Source: CAD feature listing. Evaluate the final solid. Frame: model axes, mm. Face numbers are marked on the shaded views. A direction names the side the tool comes from. Round coordinates to 2 decimals unless told otherwise and drop trailing zeros. Loops run counter-clockwise (first coordinate to the right, second up) from the corner with the lowest first, then second, coordinate; pieces in that order, holes last. Notation, with made-up numbers: (78.5, -1.75) -> (130.5, -1.75) arc R34 cw to (130.5, 28.25) -> close; hole circle Ø5 at (2, -6). An arc over 180 degrees is marked (long way). Write item = value, one per line.
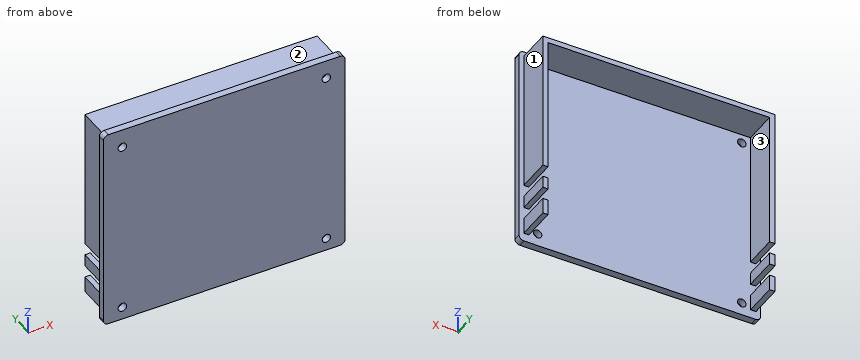
Autodesk Inventor part; units mm, degrees
ref_plane "YZ Plane" through (0, 0, 0) normal (1, 0, 0) x (0, 1, 0)
ref_plane "XZ Plane" through (0, 0, 0) normal (0, 1, 0) x (-1, 0, 0)
ref_plane "XY Plane" through (0, 0, 0) normal (0, 0, 1) x (1, 0, 0)
sketch "Sketch1" plane through (0, 0, 0) normal (0, 1, 0) x (-1, 0, 0)
  line L0 (0, 0) -> (100, 0)
  line L1 (100, 0) -> (100, -85)
  line L2 (100, -85) -> (0, -85)
  line L3 (0, -85) -> (0, 0)
  line L4 (100, -85) -> (100, -81.5)
  line L5 (100, -85) -> (0, -85)
  line L6 (0, 0) -> (100, 0)
  dimension "d0" = 100
  dimension "d1" = 85
extrude "Extrusion1" add sketch "Sketch1" along normal blind 3
sketch "Sketch5" plane through (0, 3, 0) normal (0, 1, 0) x (1, 0, 0)
  line L0 (-100, 85.001914) -> (0, 85.001914)
  line L1 (0, 85.001914) -> (0, 0.001914)
  line L2 (0, 0.001914) -> (-100, 0.001914)
  line L3 (0, 0.001914) -> (0, 3.501877)
  line L4 (0, 0.001914) -> (-100, 0.001914)
  line L5 (-100, 85.001914) -> (0, 85.001914)
  line L6 (-100, 85) -> (-100, 0)
  line L7 (-100, 85) -> (-100, 0)
  line L8 (0, 81.501879) -> (-13.977379, 81.501879)
  line L9 (0, 85) -> (-100, 85)
  line L10 (-13.977379, 81.501879) -> (-13.977379, 85)
  line L11 (0, 0) -> (0, 85)
  line L12 (0, 81.501879) -> (0, 85)
  line L13 (0, 85) -> (-13.977379, 85)
  line L14 (0, 81.501879) -> (-6, 81.501879)
  line L15 (-100, 85) -> (-100, 0)
  line L16 (-100, 0) -> (0, 0)
  line L17 (-100, 81.501917) -> (-84.168275, 81.501917)
  line L18 (-84.168275, 85) -> (-84.168275, 81.501917)
  line L19 (-93.931804, 81.467894) -> (-95.682804, 81.467894)
  line L20 (-98.248671, 81.501917) -> (-100, 81.501917)
  line L21 (-47.950989, 85) -> (-11.964435, 85)
  line L22 (-57.205258, 85) -> (-86.408023, 85)
  circle A0 centre (-7.75, 7.751877) radius 1.75
  circle A1 centre (-92.181804, 7.751877) radius 1.75
  circle A2 centre (-7.724421, 79.777458) radius 1.724421
  circle A3 centre (-92.171647, 79.74176) radius 1.760157
  line L23 (-6, 6.035046) -> (-6, 6.001877)
  line L24 (-1.751121, 81.501879) -> (-1.951121, 81.501879)
  line L25 (-1.951121, 81.501879) -> (-1.951121, 1.951914)
  line L26 (-98.048671, 1.951914) -> (-98.048671, 81.501917)
  line L27 (-98.048671, 1.951914) -> (-1.951121, 1.951914)
  line L28 (-4.180804, 81.501879) -> (-4.080804, 81.501879)
  line L29 (-4.080804, 81.501879) -> (-4.080804, 4.116343)
  line L30 (-95.682804, 81.501917) -> (-95.782804, 81.501917)
  line L31 (-95.782804, 81.501917) -> (-95.782804, 4.116343)
  line L32 (-95.782804, 4.116343) -> (-4.080804, 4.116343)
  line L33 (0, 85) -> (0, 75)
  line L34 (-1.951121, 75) -> (-4.080804, 75)
  line L35 (-4.080804, 75) -> (-4.080804, 70)
  line L36 (-4.080804, 70) -> (-1.951121, 70)
  line L37 (-1.951121, 70) -> (-1.951121, 65)
  line L38 (-1.951121, 65) -> (-4.080804, 65)
  line L39 (-4.080804, 65) -> (-4.080804, 60)
  line L40 (-4.080804, 60) -> (-1.951121, 60)
  line L41 (-95.782804, 60) -> (-98.048671, 60)
  line L42 (-95.782804, 65) -> (-98.048671, 65)
  line L43 (-95.782804, 70) -> (-98.048671, 70)
  line L44 (-95.782804, 75) -> (-98.048671, 75)
  point P0 (-92.171647, 81.501917)
  point P1 (-7.724421, 81.501879)
  dimension "d22" = 100
  dimension "d23" = 85
  dimension "d61" = 3.5
  dimension "d74" = 0.1
extrude "Extrusion10" add sketch "Sketch5" along normal blind 14 contours L17 L31 L44 L26 | L43 L31 L42 L26 | L41 L31 L32 L29 L40 L25 L27 L26 | L25 L34 L29 L8 | L25 L38 L29 L36
extrude "Extrusion11" cut sketch "Sketch5" against normal through all contours A3 | A2 | A0 | A1
fillet "Fillet1" radius 2 4 edges at (-100, 1.5, -85) (-100, 1.5, 0) (0, 1.5, -85) (0, 1.5, 0)
1. Section query A-A (y = 11.5). Return the cut outline in (x, z), then the cut area to 3 significant figures.
Evaluation:
outline = (-98.05, -81.5) -> (-95.78, -81.5) -> (-95.78, -75) -> (-98.05, -75) -> close; (-98.05, -70) -> (-95.78, -70) -> (-95.78, -65) -> (-98.05, -65) -> close; (-98.05, -60) -> (-95.78, -60) -> (-95.78, -4.12) -> (-4.08, -4.12) -> (-4.08, -60) -> (-1.95, -60) -> (-1.95, -1.95) -> (-98.05, -1.95) -> close; (-4.08, -81.5) -> (-1.95, -81.5) -> (-1.95, -75) -> (-4.08, -75) -> close; (-4.08, -70) -> (-1.95, -70) -> (-1.95, -65) -> (-4.08, -65) -> close
area = 504 mm²
2. Contact query for flat-ended pins moving along their axis: pin 1 Ø5 at (x, z) = (-45.5, -45.5) entering from -Y; pin 2 Ø1.8 at (x, y) = (-96.5, 9.5) entering from +Z; pin 3 Ø3 at (x, y) = (-25, 14.5) entering from -Z; pin 4 Ø4 at (y, z) = (8.5, -67.5) entering from +X. Output: stop coordinate, or through.
Evaluation:
pin_1 = 0
pin_2 = -1.95
pin_3 = -4.12
pin_4 = -1.95
3. Section query D-D (x = -33.5). Return the cut outline in (y, z), then the cut area to 3 significant figures.
Evaluation:
outline = (0, -85) -> (3, -85) -> (3, -4.12) -> (17, -4.12) -> (17, -1.95) -> (3, -1.95) -> (3, 0) -> (0, 0) -> close
area = 285 mm²
4. Section query B-B (x = -7.75). Return the cut outline in (y, z), then the cut area to 3 significant figures.
Evaluation:
outline = (0, -85) -> (3, -85) -> (3, -81.5) -> (0, -81.5) -> close; (0, -78.05) -> (3, -78.05) -> (3, -9.5) -> (0, -9.5) -> close; (0, -6) -> (3, -6) -> (3, -4.12) -> (17, -4.12) -> (17, -1.95) -> (3, -1.95) -> (3, 0) -> (0, 0) -> close
area = 264 mm²
5. Line query: probe 1 along X at (y, z) = (10, -19); probe 2 along X at (y, z) = (2.5, -79); probe 3 along Y at (x, z) = (-17.5, -41). Output: solid intervals per line, ascending. Write a range as from..to.
Evaluation:
probe_1 = -98.05..-95.78, -4.08..-1.95
probe_2 = -100..-93.77, -90.58..-9.26, -6.19..0
probe_3 = 0..3
6. Set-up query: the marked faces 1, 2 and 3. Return all of +Z, -Z, +X, -X, +Y, -Y with unobstructed straight access to the full face (end or side cutting, diameter ignored); none if empty.
Evaluation:
face_1 = +Z, -Z, +X, +Y
face_2 = +Z, +X, -X, +Y
face_3 = -Z, +Y
7. Section query C-C (z = -48.5). Return the cut outline in (x, y), then the cut area to 3 significant figures.
Evaluation:
outline = (-100, 0) -> (0, 0) -> (0, 3) -> (-1.95, 3) -> (-1.95, 17) -> (-4.08, 17) -> (-4.08, 3) -> (-95.78, 3) -> (-95.78, 17) -> (-98.05, 17) -> (-98.05, 3) -> (-100, 3) -> close
area = 362 mm²
